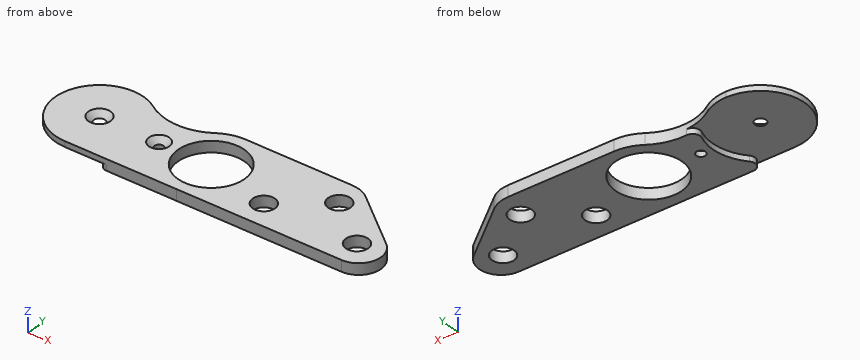
Autodesk Inventor part; units mm, degrees
ref_plane "YZ Plane" through (0, 0, 0) normal (1, 0, 0) x (0, 1, 0)
ref_plane "XZ Plane" through (0, 0, 0) normal (0, 1, 0) x (-1, 0, 0)
ref_plane "XY Plane" through (0, 0, 0) normal (0, 0, 1) x (1, 0, 0)
sketch "スケッチ1" plane through (0, 0, 0) normal (0, 0, 1) x (1, 0, 0)
  line L0 (0, 0) -> (30, 0) construction
  line L1 (0, 12) -> (30.0122, 12)
  line L2 (30, -12) -> (0, -12)
  arc A0 (0, 12) -> (0, -12) centre (0, 0) ccw
  arc A1 (30, -12) -> (30.0122, 12) centre (30, 0) ccw
  circle A2 centre (0, 0) radius 1.5
  circle A3 centre (30, 0) radius 9.025
  arc A4 (6.6694, 9.9759) -> (23.3428, 9.9759) centre (15.0061, 22.4459) ccw
  arc A5 (30.0122, 12) -> (30, -12) centre (30.0122, 0) ccw construction
  arc A6 (0, -12) -> (0, 12) centre (0, 0) ccw construction
  arc A7 (6.6694, 9.9759) -> (0, 12) centre (0, 0) ccw
  arc A8 (30.0122, 12) -> (23.3428, 9.9759) centre (30.0122, 0) ccw
  line L3 (30.0122, 12) -> (92.8308, 12)
  line L4 (92.8308, 12) -> (92.8308, -12)
  line L5 (92.8308, -12) -> (30.0122, -12)
  line L6 (30.0122, -12) -> (30.0122, 12)
  circle A9 centre (16, 0) radius 1.25
  point P0 (30.0122, -12)
  dimension "d0" = 30
  dimension "d1" = 12
  dimension "d2" = 3
  dimension "d3" = 18.05
  dimension "d6" = 15
  dimension "d11" = 2.5
  dimension "d12" = 16
extrude "押し出し1" add sketch "スケッチ1" along normal blind 3 contours A7 A4 A8 L6 A3 A1 L2 A0 | L3 L4 L5 A1 | A1 L6 A3
sketch "スケッチ2" plane through (0, 0, 0) normal (0, 0, -1) x (-1, 0, 0)
  arc A0 (-30.0122, -12) -> (-30, -12) centre (-30, 0) ccw
  line L0 (-92.8308, 12) -> (-30.0122, 12)
  line L1 (-92.8308, -12) -> (-92.8308, 12)
  line L2 (0, -12) -> (-30, -12)
  arc A1 (0, -12) -> (-6.6694, 9.9759) centre (0, 0) ccw
  arc A2 (-23.3428, 9.9759) -> (-6.6694, 9.9759) centre (-15.0061, 22.4459) ccw
  circle A3 centre (0, 0) radius 1.5
  circle A4 centre (-30, 0) radius 9.025
  arc A5 (-23.3428, 9.9759) -> (-6.6694, 9.9759) centre (-15.0061, 22.4459) ccw
  arc A6 (-6.6694, 9.9759) -> (0, -12) centre (0, 0) ccw
  arc A7 (-7.8, 10.4) -> (0, -13) centre (0, 0) ccw
  line L3 (-30.0122, -12) -> (-92.8308, -12)
  arc A8 (-23.3428, 9.9759) -> (-30.0122, 12) centre (-30.0122, 0) ccw
  point P0 (-9.9986, 8.3083)
  point P1 (-5, -12)
  point P2 (-10.0009, 8.3056)
  dimension "d7" = 1
extrude "押し出し2" cut sketch "スケッチ2" against normal blind 1.5 contours A7 A2 A6 L2 | A6 A1
fillet "フィレット1" radius 2 2 edges at (10.0009, 8.3056, 0.75) (5, -12, 0.75)
sketch "スケッチ3" plane through (0, 0, 3) normal (0, 0, 1) x (1, 0, 0)
  line L0 (92.8308, 12) -> (30.0122, 12)
  arc A0 (30.0122, 12) -> (23.3428, 9.9759) centre (30.0122, 0) ccw
  arc A1 (6.6694, 9.9759) -> (23.3428, 9.9759) centre (15.0061, 22.4459) ccw
  arc A2 (6.6694, 9.9759) -> (0, -12) centre (0, 0) ccw
  line L1 (0, -12) -> (30, -12)
  arc A3 (30, -12) -> (30.0122, -12) centre (30, 0) ccw
  line L2 (30.0122, -12) -> (92.8308, -12)
  line L3 (92.8308, -12) -> (92.8308, 12)
  circle A4 centre (30, 0) radius 9.025
  circle A5 centre (0, 0) radius 1.5
  circle A6 centre (16, 0) radius 1.25
  circle A7 centre (48, -5) radius 3.025
  circle A8 centre (73, -5) radius 3.025
  circle A9 centre (60.5, 5) radius 3.025
  line L4 (48, -5) -> (73, -5) construction
  line L5 (92.8308, 12) -> (30.0122, 12)
  line L6 (61.3547, 12) -> (92.8308, -13.1809)
  line L7 (92.8308, -12) -> (92.8308, 12)
  line L8 (60.5, 5) -> (73, -5) construction
  line L9 (60.5, 5) -> (60.5, -5) construction
  point P0 (60.5, 0)
  point P1 (91.3547, -12)
  dimension "d13" = 6.05
  dimension "d14" = 6.05
  dimension "d15" = 6.05
  dimension "d16" = 25
  dimension "d17" = 10
  dimension "d18" = 18
  dimension "d19" = 6
extrude "押し出し3" cut sketch "スケッチ3" against normal blind 10 contours L3 L2 L6 L0 | A7 | A8 | A9
fillet "フィレット2" radius 8 1 edges at (61.3547, 12, 1.5)
fillet "フィレット3" radius 6 1 edges at (91.3547, -12, 1.5)
chamfer "面取り1" distance 1.5 angle 45 2 edges at (-1.5, 0, 3) (14.75, 0, 3)
properties part number "揺動節左"
Could you check a few things on this model? Use its own coordinates, in mm. Round coordinates to 2 decimals unless told otherwise and drop trailing zeros. Loops run counter-clockwise (first coordinate to the right, second up) from the corner with the lowest first, then second, coordinate; pieces in that order, holes last. Notation, with made-up numbers: (20.25, 67) - (71.25, 67) arc R20 ccw to (71.25, 73) - close; hole circle Ø10 at (50, 12). An arc over 180 degrees is marked (long way). Use CSV: the item, a comma, the result in double quotes.
Item 1: If we section it at B-B on x = 60.5: List the corners of the cut face in (y, z) for me (3 decimals), then the cut area to 3 significant figures.
Here are the results:
outline,"(-12, 0) - (1.975, 0) - (1.975, 3) - (-12, 3) - close; (8.025, 0) - (11.758, 0) - (11.758, 3) - (8.025, 3) - close"
area,"53.1 mm²"
Item 2: Will these pins go through, and if not, where does the flat tip stop? pin 1 (3 mm diameter, centred on x = 16, y = 0, fed in from +Z); pin 2 (7 mm diameter, centred on x = 3.5, y = 2, fed in from -Z); pin 3 (5 mm diameter, centred on x = 25, y = 6.5, fed in from -Z); pin 4 (3.5 mm diameter, centred on x = 73, y = -5, fed in from +Z).
Here are the results:
pin 1,"stops at z = 1.75"
pin 2,"stops at z = 1.5"
pin 3,"stops at z = 0"
pin 4,"passes through"
Item 3: If we section it at D-D on x = 16: List the corners of the cut face in (y, z) for me.
Here are the results:
outline,"(-12, 0) - (-1.25, 0) - (-1.25, 1.5) - (-2.75, 3) - (-12, 3) - close; (1.25, 0) - (7.48, 0) - (7.48, 3) - (2.75, 3) - (1.25, 1.5) - close"
Item 4: If we section it at A-A on y = 0: Count the separate pieces of the cut face and the enclosed holes in it, then the cut area to 3 significant figures.
Here are the results:
separate pieces,"4"
enclosed holes,"0"
area,"157 mm²"
Item 5: I need wall thicknesses on L1, parallel to Y at x = 48, z = 1.75 (3 decimals); L2, parallel to Y at x = 16, z = 0.8; L3, parallel to X at y = 0, z = 1.8 (3 decimals). Which ranges of each line are inside material? Lowest first, please. Write a range as [from, to].
Here are the results:
L1,"y = [-12, -8.025], [-1.975, 12]"
L2,"y = [-12, -1.25], [1.25, 7.48]"
L3,"x = [-12, -1.8], [1.8, 14.45], [17.55, 20.975], [39.025, 76.355]"
